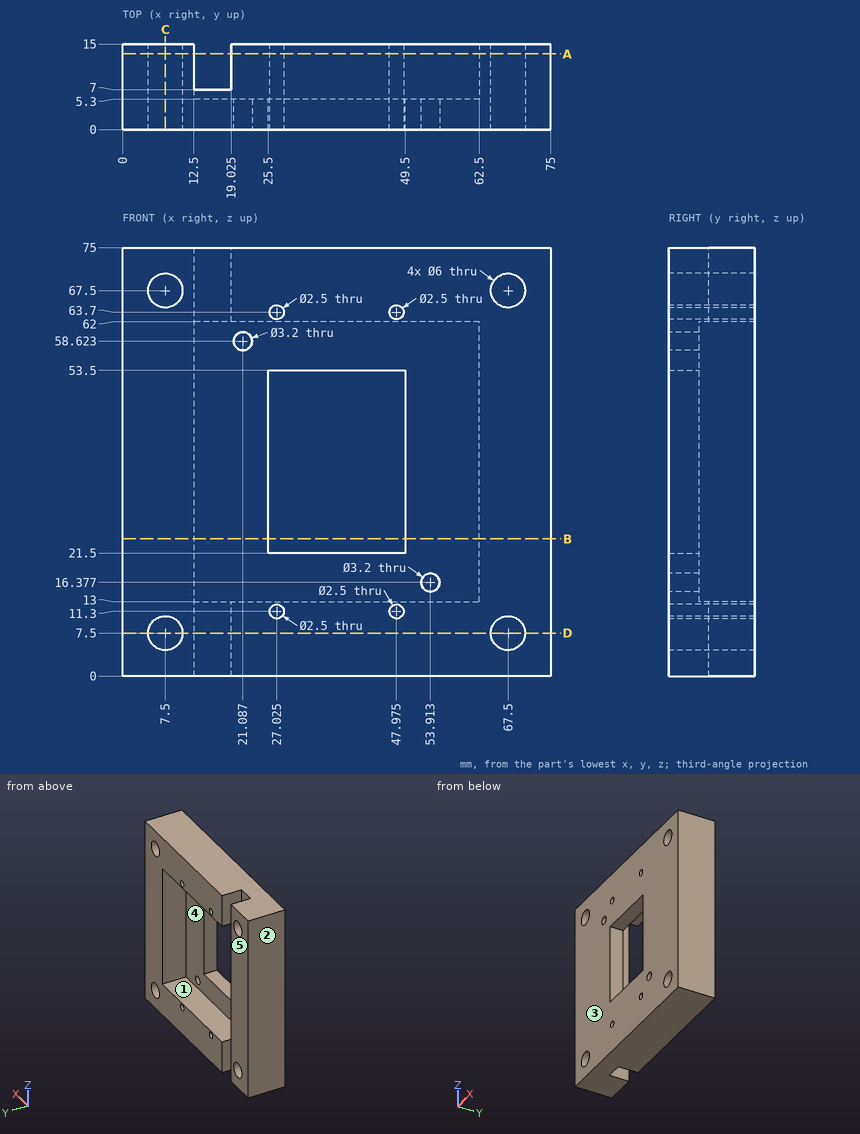
For this review, use the dimensioned drawing (mm, ordinates from the lowest corner) and the shaded views. A direction names the side the tool comes from. Round coordinates to 2 decimals unless told otherwise and drop trailing zeros. Write each loop counter-clockwise with the first axis right and the second up, starting at its lowest first coordinate (ties: lowest second). Pieces come first, ordered by that corner, then holes. Notation, with made-up numbers: M -27.5,-31 L 14.5,-31 A16 cw 14.5,-2 Z; hole C 33,22.5 d2. An arc over 180 degrees is marked long. Answer as CSV lines item,"result". Start each with the question number.
Q1. Tool access review of the marked faces 4 and 5: name each direction out of +Z, -Z, +X, -X, +Y, -Y from which nothing blocks a thin tool from reaching the whole face with its end or side.
Q2. Clearance check with flat-ended pins moving along their axes: P1, Ø4, axis at x = 47.975, z = 63.7, coming from the -Y side; P2, Ø2.5, axis at x = 21.09, z = 58.62, coming from the -Y side. State where each tip first meets the part, or that it passes through.
Q3. Wall thickness on line 1 along Z through (x, y) = (67.5, 11.25); line 2 along X through (y, z) = (0.75, 29); line 3 along X through (y, z) = (8.5, 60.5): over which ranges is each line inside the solid? List them lowest first.
Q4. The part is to be moulded in two halves that separate along X. For the marked faces 1, 2 and 3, say which applies: +X half, -X half, draft (parallel to the pull), parting line (faces both ways), or undercut.
Q5. Consider section C-C, the plane x = 7.5. Give the boundary of the cut face in (y, z), then the cut area to 3 significant figures.
Q6. Consider section A-A, the plane y = 13.25. State how many separate pieces and enclosed holes the cut face has, then the cut area to 3 significant figures.
Q7. Consider section D-D, the plane z = 7.5. Give the boundary of the cut face in (x, y) (3 decimals), then the cut area to 3 significant figures.
Q8. Consider section B-B, the plane z = 24. Give the boundary of the cut face in (x, y).
Result set:
1,face 4,"+Y"
1,face 5,"+Z, -Z, +X, -X, +Y"
2,P1,"stops at y = 0"
2,P2,"passes through"
3,line 1,"z = 0 to 4.5, 10.5 to 64.5, 70.5 to 75"
3,line 2,"x = 0 to 25.5, 49.5 to 75"
3,line 3,"x = 0 to 12.5, 62.5 to 75"
4,face 1,"undercut"
4,face 2,"-X half"
4,face 3,"draft"
5,outline,"M 0,0 L 15,0 L 15,4.5 L 0,4.5 Z; M 0,10.5 L 15,10.5 L 15,64.5 L 0,64.5 Z; M 0,70.5 L 15,70.5 L 15,75 L 0,75 Z"
5,area,"945 mm²"
6,separate pieces,"2"
6,enclosed holes,"8"
6,area,"2,870 mm²"
7,outline,"M 0,0 L 4.5,0 L 4.5,15 L 0,15 Z; M 10.5,0 L 64.5,0 L 64.5,15 L 19.025,15 L 19.025,7 L 12.5,7 L 12.5,15 L 10.5,15 Z; M 70.5,0 L 75,0 L 75,15 L 70.5,15 Z"
7,area,"893 mm²"
8,outline,"M 0,0 L 25.5,0 L 25.5,5.3 L 12.5,5.3 L 12.5,15 L 0,15 Z; M 49.5,0 L 75,0 L 75,15 L 62.5,15 L 62.5,5.3 L 49.5,5.3 Z"
